Can you work these out from the model? Positions are in its coordinate system, mm. Face numbers are marked on the shaded views. Give positions to 0.01 mm unless a question says otherwise; leave off trailing zeros. Loops run counter-clockwise (first coordinate to the right, second up) from the corner with the lowest first, then second, coordinate; pieces in that order, holes last. Notation, with made-up numbers: M 51.25,3.5 L 99.25,3.5 A12 ccw 99.25,18.5 Z; hole C -11.75,-29.5 d4. An arc over 180 degrees is marked long. One line per item, written item: value. Start each with the question number.
from build123d import *

# Parameters (mm, degrees)
SKETCH_W     = 60
SKETCH_H     = 60
PAD_DEPTH    = 3
SKETCH001_W  = 54
SKETCH001_H  = 54
PAD001_DEPTH = 3
SKETCH002_R  = 3.5
PAD002_DEPTH = 6
SKETCH003_R  = 2
POCKET_DEPTH = 8


with BuildPart() as part:
    # Sketch → Pad (new body)
    with BuildSketch(Plane.XY):
        Rectangle(SKETCH_W, SKETCH_H)
    extrude(amount=PAD_DEPTH)

    # Sketch001 (on Face6 of Pad) → Pad001 (join)
    with BuildSketch(Plane.XY.offset(3)):
        Rectangle(SKETCH001_W, SKETCH001_H)
    extrude(amount=PAD001_DEPTH)

    # Sketch002 (on Face11 of Pad001) → Pad002 (join)
    with BuildSketch(Plane.XY.offset(6)):
        with Locations((-20.32, 20.32)):
            Circle(SKETCH002_R)
        with Locations((20.32, 20.32)):
            Circle(SKETCH002_R)
        with Locations((20.32, -20.32)):
            Circle(SKETCH002_R)
        with Locations((-20.32, -20.32)):
            Circle(SKETCH002_R)
    extrude(amount=PAD002_DEPTH)

    # Sketch003 (on Face19 of Pad002) → Pocket (cut)
    with BuildSketch(Plane.XY.offset(12)):
        with Locations((-20.32, 20.32)):
            Circle(SKETCH003_R)
        with Locations((20.32, 20.32)):
            Circle(SKETCH003_R)
        with Locations((20.32, -20.32)):
            Circle(SKETCH003_R)
        with Locations((-20.32, -20.32)):
            Circle(SKETCH003_R)
    extrude(amount=-POCKET_DEPTH, mode=Mode.SUBTRACT)


solid = part.part
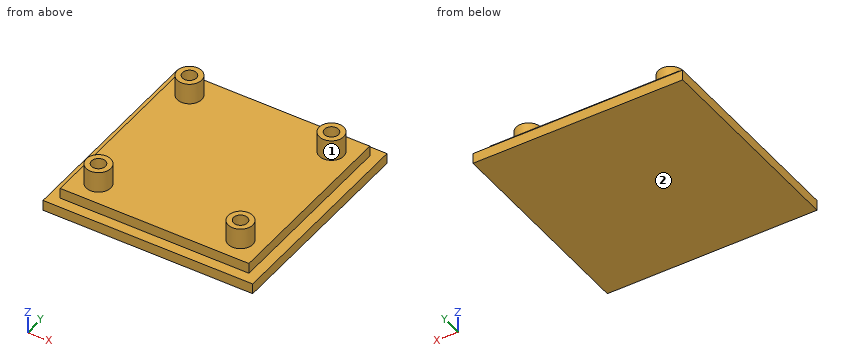
Q1. I need wall thicknesses on line 1 along Y through (x, z) = (-20.32, 6.5); line 2 along Z through (x, y) = (6, 5); line 3 along X through (y, z) = (0, 3.5). Which ranges of each line are inside material? Lowest first, please.
Q2. If we section it at C-C, the plane y = 20.32: Write out the boundary of the cut face in (x, z).
Q3. If we section it at A-A, the plane x = -12.5: Write out the boundary of the cut face in (y, z).
Q4. If we mould it in two halves opening along X, with no side actions, what happens to the marked faces 1 and 2? For each: released by +X, released by -X, zero draft, split by the parting line, or undercut.
Q5. For P1, Ø1.5, axis at y = -12, z = 4, coming from the -X side; P2, Ø18, axis at x = -2.5, y = 12, coming from the +Z side; P3, Ø2, axis at x = 19, z = 10.5, coming from the +Y side, each with a flat end and sliding along its axis, tell me the tip position at first contact or that it passes through.
Response:
1. line 1: -23.82 to -22.32, -18.32 to -16.82, 16.82 to 18.32, 22.32 to 23.82
1. line 2: 0 to 6
1. line 3: -27 to 27
2. outline: M -30,0 L 30,0 L 30,3 L 27,3 L 27,6 L 23.82,6 L 23.82,12 L 22.32,12 L 22.32,4 L 18.32,4 L 18.32,12 L 16.82,12 L 16.82,6 L -16.82,6 L -16.82,12 L -18.32,12 L -18.32,4 L -22.32,4 L -22.32,12 L -23.82,12 L -23.82,6 L -27,6 L -27,3 L -30,3 Z
3. outline: M -30,0 L 30,0 L 30,3 L 27,3 L 27,6 L -27,6 L -27,3 L -30,3 Z
4. face 1: undercut
4. face 2: zero draft
5. P1: x = -27
5. P2: z = 6
5. P3: y = 23.81
